Job drawing, mm, ordinate dimensions from the low corner. One solid piece. Round coordinates to 2 decimals unless told otherwise and drop trailing zeros. Loops run counter-clockwise (first coordinate to the right, second up) from the corner with the lowest first, then second, coordinate; pieces in that order, holes last.
1) Band-saw the part on D-D, the plane z = 13.5. Write the cut outline in (x, y).
2) Mould opens along X. For the marked faces 1 and 2 say: +X half, -X half, draft (parallel to the pull), parting line (faces both ways), or undercut.
3) Band-saw the part on B-B, the plane z = 39. Write the cut outline in (x, y), then the cut area to 3 significant figures.
4) Probe line 1 (Y direction, x = 95, z = 6); line 2 (Y direction, x = 164, z = 6); line 3 (Y direction, x = 95, z = 45). List the from-to ranges inside material, lowest first.
5) Drop flat-ended pins along their axis: P1, Ø3.5, axis at x = 163, z = 38, coming from the +Y side; P2, Ø3.5, axis at x = 26, z = 39, coming from the -Y side; P3, Ø4, axis at x = 156, z = 40, coming from the +Y side. Give the stop position or say it passes through.
6) Band-saw the part on A-A, the plane y = 95. Write the cut outline in (x, z).
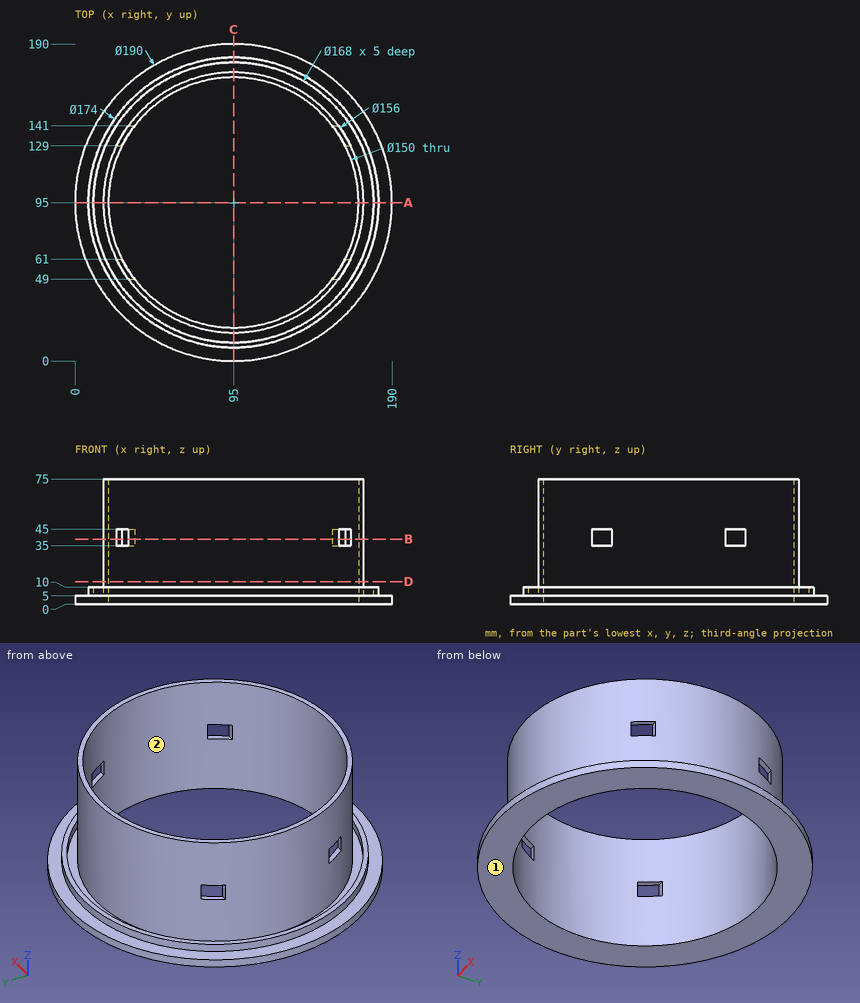
Reported:
1. outline: circle Ø156 at (95, 95); hole circle Ø150 at (95, 95)
2. face 1: draft
2. face 2: undercut
3. outline: (24.8, 61) - (28.15, 61) arc R75 cw to (28.15, 129) - (24.8, 129) arc R78 ccw to start; (32.01, 49) arc R78 ccw to (157.99, 49) - (154.24, 49) arc R75 cw to (35.76, 49) - close; (32.01, 141) - (35.76, 141) arc R75 cw to (154.24, 141) - (157.99, 141) arc R78 ccw to start; (161.85, 61) - (165.2, 61) arc R78 ccw to (165.2, 129) - (161.85, 129) arc R75 cw to start
3. area: 1,270 mm2
4. line 1: y = 8 to 11, 17 to 20, 170 to 173, 179 to 182
4. line 2: y = 42.01 to 47.09, 58.63 to 65.61, 124.39 to 131.37, 142.91 to 147.99
4. line 3: y = 17 to 20, 170 to 173
5. P1: stops at y = 129
5. P2: stops at y = 61
5. P3: stops at y = 146.02
6. outline: (0, 0) - (20, 0) - (20, 75) - (17, 75) - (17, 5) - (11, 5) - (11, 10) - (8, 10) - (8, 5) - (0, 5) - close; (170, 0) - (190, 0) - (190, 5) - (182, 5) - (182, 10) - (179, 10) - (179, 5) - (173, 5) - (173, 75) - (170, 75) - close
